Design review of the part built by this model. Coordinates are the model's own, in mm. Coordinates: 2 decimals unless noted, no trailing zeros. Write each loop counter-clockwise with the first axis right and the second up, starting at its lowest first coordinate (ties: lowest second). Pieces come first, ordered by that corner, then holes. Notation, with made-up numbers: (-12, 72) - (15, 72) arc R23 ccw to (15, 109) - close; hole circle Ø7 at (17, 32). An arc over 180 degrees is marked (long way). Use a Markdown table: item, result.
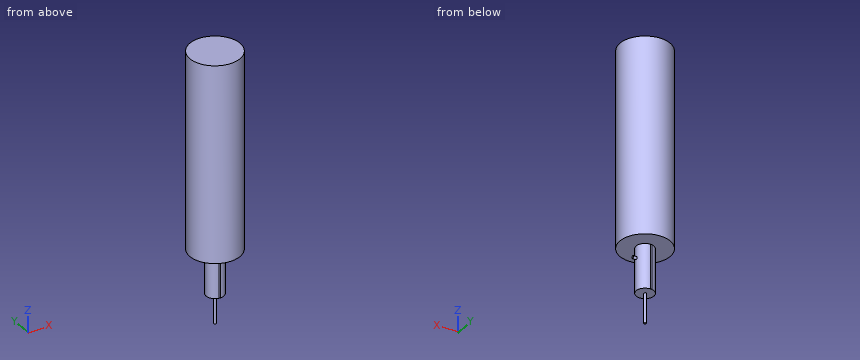
from build123d import *
from build123d.topology import SkipClean

# Parameters (mm, degrees)
ESQUISSE1_R             = 11.35
BOSS_EXTRU_1_DEPTH      = 88.5
ESQUISSE2_R             = 4
BOSS_EXTRU_2_DEPTH      = 20
ESQUISSE4_W             = 0.590657656
ESQUISSE4_H             = 10.980800687
BOSS_EXTRU_3_DEPTH      = 20
ESQUISSE5_R             = 0.615112373
BOSS_EXTRU_4_DEPTH      = 5.6
ENL_V_START             = -20
ENL_V_MAT_EXTRU_2_DEPTH = 20
ENL_V_MAT_EXTRU_3_DEPTH = 20
SKETCH1_R               = 0.5
BOSS_EXTRUDE1_DEPTH     = 13.4


with BuildPart() as part:
    # Esquisse1 → Boss.-Extru.1 (new body)
    with BuildSketch(Plane.XY):
        Circle(ESQUISSE1_R)
    extrude(amount=BOSS_EXTRU_1_DEPTH)

    # Esquisse2 → Boss.-Extru.2 (add)
    with BuildSketch(Plane(origin=(0, 0, 0), x_dir=(-1, 0, 0), z_dir=(0, 0, -1))):
        Circle(ESQUISSE2_R)
    extrude(amount=BOSS_EXTRU_2_DEPTH)

    # Esquisse4 → Boss.-Extru.3 (add)
    with BuildSketch(Plane(origin=(0, 0, 0), x_dir=(-1, 0, 0), z_dir=(0, 0, -1))):
        with Locations((0.295328828, 1.490400344)):
            Rectangle(ESQUISSE4_W, ESQUISSE4_H)
    extrude(amount=BOSS_EXTRU_3_DEPTH)

    # Esquisse5 → Boss.-Extru.4 (add)
    with BuildSketch(Plane(origin=(0, 0, 0), x_dir=(0, 0, -1), z_dir=(1, 0, 0))):
        with Locations((5.5, 0)):
            Circle(ESQUISSE5_R)
    extrude(amount=BOSS_EXTRU_4_DEPTH)

    # Esquisse7 → Enlèv. mat.-Extru.2 (cut)
    with BuildSketch(Plane(origin=(0, 0, -20), x_dir=(-1, 0, 0), z_dir=(0, 0, -1)).offset(ENL_V_START)):
        with BuildLine():
            Line((0.590657656, 6.980800687), (0, 6.980800687))
            Line((0, 6.980800687), (0, 4))
            ThreePointArc((0, 4), (0.296141555, 3.989022459), (0.590657656, 3.95615009))
            Line((0.590657656, 3.95615009), (0.590657656, 6.980800687))
        make_face()
    extrude(amount=ENL_V_MAT_EXTRU_2_DEPTH, mode=Mode.SUBTRACT)

    # Esquisse8 → Enlèv. mat.-Extru.3 (cut)
    with SkipClean():  # the faces are left unmerged after this step: merging them gives an invalid solid
        with BuildSketch(Plane(origin=(0, 0, -20), x_dir=(-1, 0, 0), z_dir=(0, 0, -1)).offset(ENL_V_START)):
            with BuildLine():
                ThreePointArc((0.590657656, -3.95615009), (0.296141555, -3.989022459), (0, -4))
                Line((0, -4), (0.590657656, -4))
                Line((0.590657656, -4), (0.590657656, -3.95615009))
            make_face()
        extrude(amount=ENL_V_MAT_EXTRU_3_DEPTH, mode=Mode.SUBTRACT)

    # Sketch1 → Boss-Extrude1 (add)
    with SkipClean():  # the faces are left unmerged after this step: merging them gives an invalid solid
        with BuildSketch(Plane(origin=(0, 0, -20), x_dir=(-1, 0, 0), z_dir=(0, 0, -1))):
            Circle(SKETCH1_R)
        extrude(amount=BOSS_EXTRUDE1_DEPTH)


solid = part.part
(1) Take a section at D-D on z = -8. Write out the cut boundary in (x, y).
Determined:
| item | result |
|---|---|
| outline | circle Ø8 at (0, 0) |
(2) Take a section at A-A on z = 55. Write out the cut boundary in (x, y), and give its area (3 significant figures).
Determined:
| item | result |
|---|---|
| outline | circle Ø22.7 at (0, 0) |
| area | 405 mm2 |
(3) Take a section at C-C on x = -2.25. Write out the cut boundary in (y, z), and give its area (3 significant figures).
Determined:
| item | result |
|---|---|
| outline | (-11.12, 0) - (-3.31, 0) - (-3.31, -20) - (3.31, -20) - (3.31, 0) - (11.12, 0) - (11.12, 88.5) - (-11.12, 88.5) - close |
| area | 2,100 mm2 |
(4) For L1, parallel to Z at x = -7.5, y = -5.5; L2, parallel to X at y = 0.5, z = 59; L3, parallel to Y at x = -0.25, z = -8, list the stretches that pass through material, from the lowest coordinate up. Write a range as from..to.
Determined:
| item | result |
|---|---|
| L1 | 0..88.5 |
| L2 | -11.34..11.34 |
| L3 | -3.99..3.99 |
(5) For pin 1 (1 mm diameter, centred on y = 5, z = 70, fed in from +X); pin 2 (6 mm diameter, centred on y = -9, z = 65, fed in from +X); pin 3 (7 mm diameter, centred on x = 4.5, y = 0, fed in from -Z), all flat-tipped, find the tip position at first contact; note any pin that passes through.
Determined:
| item | result |
|---|---|
| pin 1 | x = 10.42 |
| pin 2 | x = 9.63 |
| pin 3 | z = -20 |
(6) Take a section at B-B on y = 1.75. Write out the cut boundary in (x, z), and give its area (3 significant figures).
Determined:
| item | result |
|---|---|
| outline | (-11.21, 0) - (-3.6, 0) - (-3.6, -20) - (3.6, -20) - (3.6, 0) - (11.21, 0) - (11.21, 88.5) - (-11.21, 88.5) - close |
| area | 2,130 mm2 |
